from build123d import *

# Parameters (mm, degrees)
ESQUISSE2_W             = 30
ESQUISSE2_H             = 84
BOSS_EXTRU_1_DEPTH      = 15
ESQUISSE3_R             = 29
ENL_V_MAT_EXTRU_1_DEPTH = 10
CHANFREIN1_SIZE         = 20
CHANFREIN1_SIZE_2       = 5
CHANFREIN2_SIZE         = 15


with BuildPart() as part:
    # Esquisse2 → Boss.-Extru.1 (new body)
    with BuildSketch(Plane(origin=(0, 0, 0), x_dir=(1, 0, 0), z_dir=(0, 1, 0))):
        with Locations((-17.412854797, -1.219560319)):
            Rectangle(ESQUISSE2_W, ESQUISSE2_H)
    extrude(amount=BOSS_EXTRU_1_DEPTH)

    # Esquisse3 → Enlèv. mat.-Extru.1 (cut)
    with BuildSketch(Plane(origin=(0, 15, 0), x_dir=(1, 0, 0), z_dir=(0, 1, 0))):
        with Locations((-37.412854797, 8.780439681)):
            Circle(ESQUISSE3_R)
    extrude(amount=-ENL_V_MAT_EXTRU_1_DEPTH, mode=Mode.SUBTRACT)

    # Chanfrein1
    # the kernel refuses this chamfer: 20, 5 mm, written as the material it takes off along each edge
    with BuildSketch(Plane(origin=(-32.412854797, 5, 71.727824028), x_dir=(0.9999563942249224, 0.00933861064031752, 0), z_dir=(0, 0, -1))) as chanfrein1_piece_1_section:
        Polygon((CHANFREIN1_SIZE * 0.999956394225, CHANFREIN1_SIZE * 0.00933861064032), (-CHANFREIN1_SIZE_2 * 0.00933861064032, CHANFREIN1_SIZE_2 * 0.999956394225), (0, 0), align=None)
    chanfrein1_piece_1 = extrude(amount=161.016527419, mode=Mode.PRIVATE)
    chanfrein1_piece_1 = chanfrein1_piece_1 & Plane(origin=(-37.412854797, 3.276810051, -8.780439681), x_dir=(1, 0, 0), z_dir=(0, 1, 0)) * Cylinder(29, 403, mode=Mode.PRIVATE)
    add(chanfrein1_piece_1, mode=Mode.SUBTRACT)

    # Chanfrein2
    chanfrein2_edges = [part.edges().sort_by_distance(p)[0] for p in [
        (-2.412854797, 7.5, -40.780439681),
    ]]
    chamfer(chanfrein2_edges, length=CHANFREIN2_SIZE)


solid = part.part
Design review of the part built by this model. Coordinates are the model's own, in mm. A direction names the side the tool comes from. Coordinates: 2 decimals unless noted, no trailing zeros. Order: outer loops, then holes, each group sorted by start corner. A loop starts at its lowest first (then second) coordinate and runs counter-clockwise, first axis right, second up. Notation, with made-up numbers: (25.5, 44.5) -> (46.5, 44.5) arc R24 ccw to (46.5, 63.5) -> close; hole circle Ø3 at (10, 26). An arc over 180 degrees is marked (long way). One line per item, written item: value.
1) To check wall thickness, follow probe 1 along Y at (x, z) = (-10.5, -12.5); probe 2 along Z at (x, y) = (-16.5, 4.25); probe 3 along Z at (x, y) = (-28, 12). State the ranges of each line that lie inside material, in increasing order. Write a range as [from, to].
Output values:
probe 1: y = [0, 5]
probe 2: z = [-39.87, -28.87], [11.31, 43.22]
probe 3: z = [-40.78, -36.21], [18.65, 43.22]
2) Machinability: for faces 1 (the face through (-22.273, 2.535, -8.381)), 2 (the face through (-25, 7, -40.78)), which of the approach directions +Z, -Z, +X, -X, +Y, -Y give a long, thin tool a straight path to every point of the face, cutting with its end or side? Answer none if there is none.
Output values:
face 1: -X, +Y
face 2: -Z, +X, -X, +Y, -Y
3) Draft analysis for pull direction Z (two halves, no side actions). For faces 3 (the face through (-8.42, 9.27, -8.21)), 4 (the face through (-32.413, 7, 32)), 5 (the face through (-18, 7, 43.22)), state which applies: +Z half, -Z half, draft (parallel to the pull), parting line (faces both ways), or undercut.
Output values:
face 3: undercut
face 4: draft
face 5: +Z half
4) We need section D-D, the plane y = 3.75. Give the boundary of the cut face in (x, z), then the cut area to 3 significant figures.
Output values:
outline: (-32.41, -40.78) -> (-17.41, -40.78) -> (-2.41, -25.78) -> (-2.41, 43.22) -> (-32.41, 43.22) -> (-32.41, 19.79) arc R29 cw to (-17.41, 12.22) -> (-17.41, -29.78) arc R29 cw to (-32.41, -37.35) -> close
area: 1,640 mm2
5) We need section A-A, the plane y = 12. Give the boundary of the cut face in (x, z).
Output values:
outline: (-32.41, -40.78) -> (-17.41, -40.78) -> (-2.41, -25.78) -> (-2.41, 43.22) -> (-32.41, 43.22) -> (-32.41, 19.79) arc R29 cw to (-32.41, -37.35) -> close
6) Clearance check with flat-ended pins moving along their axes: P1, Ø2, axis at x = -11, z = -8, coming from the +Y side; P2, Ø6, axis at x = -18.5, z = -6.5, coming from the +Y side. State where each tip first meets the part, or that it passes through.
Output values:
P1: stops at y = 5
P2: stops at y = 4.23
7) We need section B-B, the plane x = -26. Give the boundary of the cut face in (y, z).
Output values:
outline: (0, -40.78) -> (15, -40.78) -> (15, -35.44) -> (1.6, -35.44) -> (1.6, 17.88) -> (15, 17.88) -> (15, 43.22) -> (0, 43.22) -> close
8) We need section C-C, the plane z = -32. Give the boundary of the cut face in (x, y).
Output values:
outline: (-32.41, 0) -> (-8.63, 0) -> (-8.63, 15) -> (-20.04, 15) -> (-20.04, 3.09) -> close
